Model file for the job. Use its own axes, mm. A direction names the side the tool comes from. Coordinates: 2 decimals unless noted, no trailing zeros. Loops run counter-clockwise (first coordinate to the right, second up) from the corner with the lowest first, then second, coordinate; pieces in that order, holes last.
from build123d import *

# Parameters (mm, degrees)
CUT_EXTRUDE1_DEPTH      = 86.450904972
CIRPATTERN1_COUNT       = 18
CIRPATTERN1_ANGLE       = 180
CUT_EXTRUDE2_DEPTH      = 94.149359325
CUT_EXTRUDE2_DEPTH_BACK = 94.149359325
BOSS_EXTRUDE1_DEPTH     = 3.81
CUT_EXTRUDE4_DEPTH      = 100.573936521
CUT_EXTRUDE4_DEPTH_BACK = 100.573936521
SKETCH9_R               = 6.35


with BuildPart() as part:
    # Sketch2 → Revolve1 (revolve)
    with BuildSketch(Plane(origin=(0, 0, 0), x_dir=(0, 1, 0), z_dir=(0, 0, 1))):
        Polygon((0, -37.923611111), (-25.4, -37.923611111), (-25.4, 0), (-38.1, 0), (-38.1, 9.701388889), (-25.4, 9.701388889), (-25.4, 76.023611111), (0, 76.023611111), align=None)
    revolve(axis=Axis((-76.023611111, 0, 0), (1, 0, 0)))

    # Sketch3 → Cut-Extrude1 (cut, through all)
    with BuildSketch(Plane(origin=(-9.701388889, 0, 0), x_dir=(0, -1, 0), z_dir=(-1, 0, 0))):
        Polygon((0, 38.288766927), (2.54, 38.288766927), (1.27, 34.478766927), (0, 34.478766927), (-1.27, 34.478766927), (-2.54, 38.288766927), align=None)
    cut_extrude1 = extrude(amount=-CUT_EXTRUDE1_DEPTH, mode=Mode.SUBTRACT)

    # CirPattern1: Cut-Extrude1 ×18 about axis
    cirpattern1_axis = Axis((0, 0, 0), (-1, 0, 0))
    for i in range(1, CIRPATTERN1_COUNT):
        add(cut_extrude1.rotate(cirpattern1_axis, i * CIRPATTERN1_ANGLE / (CIRPATTERN1_COUNT - 1)), mode=Mode.SUBTRACT)

    # Sketch5 → Cut-Extrude2 (cut, two sides: drawn at the far end of the back side and taken through both)
    with BuildSketch(Plane(origin=(0, 0, 0), x_dir=(0, 1, 0), z_dir=(0, 0, 1)).offset(-CUT_EXTRUDE2_DEPTH_BACK)):
        Polygon((11.291183517, 76.023611111), (-25.4, 76.023611111), (-25.4, 49.536195496), align=None)
    extrude(amount=CUT_EXTRUDE2_DEPTH + CUT_EXTRUDE2_DEPTH_BACK, mode=Mode.SUBTRACT)

    # Sketch7 → Boss-Extrude1 (add, symmetric)
    with BuildSketch(Plane(origin=(0, 0, 0), x_dir=(0, 1, 0), z_dir=(0, 0, 1))):
        with BuildLine():
            Line((0, 67.872490271), (-7.374879009, 78.211791969))
            ThreePointArc((-7.374879009, 78.211791969), (-19.941931013, 80.231629124), (-21.978787639, 67.667324397))
            Line((-21.978787639, 67.667324397), (-14.376066372, 57.494388275))
            Line((-14.376066372, 57.494388275), (-7.054408242, 62.779903303))
            Line((-7.054408242, 62.779903303), (0, 67.872490271))
        make_face()
    extrude(amount=BOSS_EXTRUDE1_DEPTH, both=True)

    # Sketch9 → Cut-Extrude4 (cut, two sides: drawn at the far end of the back side and taken through both)
    with BuildSketch(Plane.XY.offset(3.81).offset(-CUT_EXTRUDE4_DEPTH_BACK)):
        with Locations((-72.929668111, -14.66969239)):
            Circle(SKETCH9_R)
    extrude(amount=CUT_EXTRUDE4_DEPTH + CUT_EXTRUDE4_DEPTH_BACK, mode=Mode.SUBTRACT)


solid = part.part
Q1. Slice it at B-B (x = -11.5). List the corners of the cut face in (y, z).
Answers:
outline: circle Ø50.8 at (0, 0)
Q2. Mould opens along Z. For faces 5 (the flat face through (-4.92, 25.77, 25.52)), 6 (the flat face through (0, -26, -1)), 7 (the flat face through (-4.92, 35.4, -8.13)) say: +Z half, -Z half, draft (parallel to the pull), parting line (faces both ways), or undercut.
Answers:
face 5: +Z half
face 6: draft
face 7: undercut
Q3. Flat gauge pins, fed straight in: P1, Ø8, axis at y = 25.5, z = 11, coming from the +X side; P2, Ø5, axis at x = -24, z = -17.5, coming from the +Y side; P3, Ø19, axis at x = -68.5, y = -8, coming from the -Z side; P4, Ø12, axis at x = -47.5, z = -8.5, coming from the +Y side. Where does each tip first touch, or does it go through?
Answers:
P1: stops at x = 37.92
P2: stops at y = 20.5
P3: stops at z = -25.4
P4: stops at y = 25.28
Q4. Drill centre lines: line 1 (X direction, y = -26.5, z = -20); line 2 (Z direction, x = -7.5, y = 23.5); line 3 (Z direction, x = -3, y = -20). Where is each one in solid material? Low to high.
Answers:
line 1: x = -9.7 to 0
line 2: z = -29.99 to -29.06, -25.23 to 25.23, 29.06 to 29.99
line 3: z = -32.43 to 32.43
Q5. Which spindle directions (+Z, -Z, +X, -X, +Y, -Y) get a long thin tool onto all of the face, cutting with end or side? Do faces 1 (the flat face through (-4.92, 33.25, 14.49)), 2 (the flat face through (-4.919, 27.792, -23.309)), 3 (the flat face through (-4.919, 1.869, -36.275)), 4 (the flat face through (-4.919, -1.869, 36.275)). Say none if no direction does.
Answers:
face 1: +X, -X
face 2: +X, -X, +Y
face 3: -Z, +X, -X
face 4: +Z, +X, -X
Q6. Slice it at C-C (y = -30). List the corners of the cut face in (x, z).
Answers:
outline: (-9.7, -23.49) - (0, -23.49) - (0, 23.49) - (-9.7, 23.49) - close
Q7. Slice it at A-A (y = -10). List the corners of the cut face in (x, z), and give its area (3 significant figures).
Answers:
outline: (-80.63, -3.81) - (-77.23, -3.81) - (-77.23, 3.81) - (-80.63, 3.81) - close; (-68.63, -3.81) - (-60.65, -3.81) - (-60.65, -23.35) - (-9.7, -23.35) - (-9.7, -36.76) - (0, -36.76) - (0, -23.35) - (37.92, -23.35) - (37.92, 23.35) - (0, 23.35) - (0, 36.76) - (-9.7, 36.76) - (-9.7, 23.35) - (-60.65, 23.35) - (-60.65, 3.81) - (-68.63, 3.81) - close
area: 4,950 mm2
Q8. Slice it at D-D (x = -56). List the corners of the cut face in (y, z), and give its area (3 significant figures).
Answers:
outline: (-16.45, -19.36) arc R25.4 ccw (long way) to (-16.45, 19.36) - close
area: 1,790 mm2
